Verification items for this drawing (mm, ordinates from the low corner). A direction names the side the tool comes from. Coordinates: 2 decimals unless noted, no trailing zeros. Loops run counter-clockwise (first coordinate to the right, second up) from the corner with the lowest first, then second, coordinate; pieces in that order, holes last. Notation, with made-up numbers: M -10,52 L 11,52 A36 ccw 11,89 Z; hole C 13.5,27.5 d5. An arc over 180 degrees is marked long. Return JSON: item names as keys, results as strings.
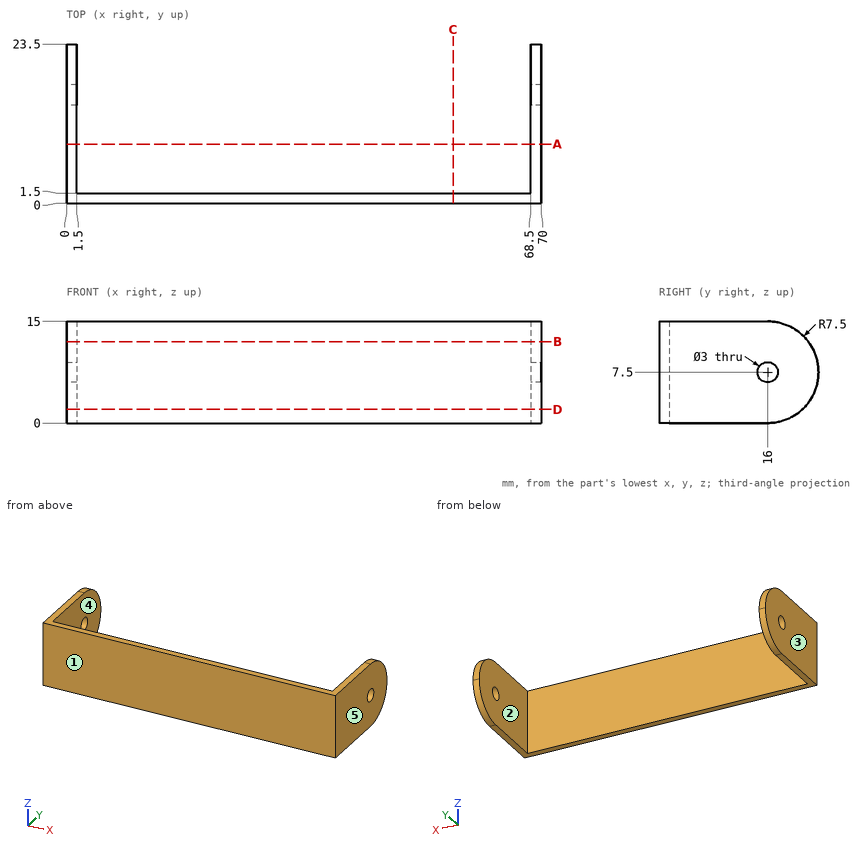
1) Go/stop test with flat-tipped pins: pin 1 Ø1.8 at (y, z) = (16, 7.5) entering from +X; pin 2 Ø1 at (x, z) = (44, 3.5) entering from +Y; pin 3 Ø8 at (x, z) = (34, 7.5) entering from -Y. Record where each tip stops, or that it passes through.
Answers:
{"pin 1": "through", "pin 2": "y = 1.5", "pin 3": "y = 0"}
2) Section check D-D on z = 2. Record the cut outline in (x, y).
Answers:
{"outline": "M 0,0 L 70,0 L 70,21.1 L 68.5,21.1 L 68.5,1.5 L 1.5,1.5 L 1.5,21.1 L 0,21.1 Z"}
3) Section check B-B on z = 12. Record the cut outline in (x, y).
Answers:
{"outline": "M 0,0 L 70,0 L 70,22 L 68.5,22 L 68.5,1.5 L 1.5,1.5 L 1.5,22 L 0,22 Z"}
4) Draft check along X on the marked faces 3, 4 and 5. Enter one of: +X half, -X half, draft (parallel to the pull), parting line (faces both ways), or undercut.
Answers:
{"face 3": "-X half", "face 4": "undercut", "face 5": "+X half"}
5) Set-up check for the marked faces 1 and 2: record each of +Z, -Z, +X, -X, +Y, -Y from which the full face is reachable in a straight line by a thin tool's end or side.
Answers:
{"face 1": "+Z, -Z, +X, -X, -Y", "face 2": "+Z, -Z, +Y"}
6) Section check C-C on x = 57. Record the cut outline in (y, z), then the cut area to 3 significant figures.
Answers:
{"outline": "M 0,0 L 1.5,0 L 1.5,15 L 0,15 Z", "area": "22.5 mm²"}
7) Scan lines: line 1 along X through (y, z) = (13.5, 13.75); line 2 along Y through (x, z) = (0.55, 7.5); line 3 along Y through (x, z) = (54, 6.75). Record each from-to range of solid material in increasing order. Write a range as [from, to].
Answers:
{"line 1": "[0, 1.5], [68.5, 70]", "line 2": "[0, 14.5], [17.5, 23.5]", "line 3": "[0, 1.5]"}
8) Section check A-A on y = 8.75. Record the cut outline in (x, z), then the cut area to 3 significant figures.
Answers:
{"outline": "M 0,0 L 1.5,0 L 1.5,15 L 0,15 Z; M 68.5,0 L 70,0 L 70,15 L 68.5,15 Z", "area": "45.0 mm²"}
